```python
from build123d import *

# Parameters (mm, degrees)
SKETCH1_W           = 9.8806
SKETCH1_H           = 5.7658
BOSS_EXTRUDE1_DEPTH = 6.985
SKETCH2_W           = 0.6604
SKETCH2_H           = 0.6604
BOSS_EXTRUDE2_DEPTH = 3.175
SKETCH4_W           = 8.6106
SKETCH4_H           = 4.4958
CUT_EXTRUDE1_DEPTH  = 6.35
SKETCH2_2_W         = 0.6604
SKETCH2_2_H         = 0.6604
BOSS_EXTRUDE3_DEPTH = 6.35
SKETCH5_W           = 0.635
SKETCH5_H           = 1.016
SKETCH5_W_2         = 1.524
SKETCH5_H_2         = 0.635
CUT_EXTRUDE2_DEPTH  = 3.556


with BuildPart() as part:
    # Sketch1 → Boss-Extrude1 (new body)
    with BuildSketch(Plane.XY):
        with Locations((4.9403, 2.8829)):
            Rectangle(SKETCH1_W, SKETCH1_H)
    extrude(amount=BOSS_EXTRUDE1_DEPTH)

    # Sketch2 → Boss-Extrude2 (add)
    with BuildSketch(Plane(origin=(0, 0, 0), x_dir=(-1, 0, 0), z_dir=(0, 0, -1))):
        with Locations((-7.4403, 3.4036)):
            Rectangle(SKETCH2_W, SKETCH2_H)
        with Locations((-4.9403, 3.4036)):
            Rectangle(SKETCH2_W, SKETCH2_H)
        with Locations((-2.4403, 3.4036)):
            Rectangle(SKETCH2_W, SKETCH2_H)
    extrude(amount=BOSS_EXTRUDE2_DEPTH)

    # Sketch4 → Cut-Extrude1 (cut)
    with BuildSketch(Plane.XY.offset(6.985)):
        with Locations((4.9403, 2.8829)):
            Rectangle(SKETCH4_W, SKETCH4_H)
    extrude(amount=-CUT_EXTRUDE1_DEPTH, mode=Mode.SUBTRACT)

    # Sketch2<2> → Boss-Extrude3 (add)
    with BuildSketch(Plane(origin=(0, 0, 0), x_dir=(-1, 0, 0), z_dir=(0, 0, -1))):
        with Locations((-7.4403, 3.4036)):
            Rectangle(SKETCH2_2_W, SKETCH2_2_H)
        with Locations((-4.9403, 3.4036)):
            Rectangle(SKETCH2_2_W, SKETCH2_2_H)
        with Locations((-2.4403, 3.4036)):
            Rectangle(SKETCH2_2_W, SKETCH2_2_H)
    extrude(amount=-BOSS_EXTRUDE3_DEPTH)

    # Sketch5 → Cut-Extrude2 (cut)
    with BuildSketch(Plane.XY.offset(6.985)):
        with Locations((0.3175, 4.3688)):
            Rectangle(SKETCH5_W, SKETCH5_H)
        with Locations((9.5631, 4.3688)):
            Rectangle(SKETCH5_W, SKETCH5_H)
        with Locations((7.2263, 5.4483)):
            Rectangle(SKETCH5_W_2, SKETCH5_H_2)
        with Locations((2.6543, 5.4483)):
            Rectangle(SKETCH5_W_2, SKETCH5_H_2)
    extrude(amount=-CUT_EXTRUDE2_DEPTH, mode=Mode.SUBTRACT)


solid = part.part
```
Geometry: final body of the model. Coordinates: model frame, mm. A direction names the side the tool comes from. Coordinates: 2 decimals unless noted, no trailing zeros. Order: outer loops, then holes, each group sorted by start corner. A loop starts at its lowest first (then second) coordinate and runs counter-clockwise, first axis right, second up. Notation, with made-up numbers: (35.25, -29.75) -> (92.25, -29.75) arc R10 ccw to (92.25, -25.75) -> close; hole circle Ø7 at (41, 33). An arc over 180 degrees is marked (long way). Write item = value, one per line.
(1) Cut plane D-D on x = 3. Return loops of the section in (y, z) (3 decimals), plus the area to 3 significant figures.
Solved:
outline = (0, 0) -> (5.766, 0) -> (5.766, 3.429) -> (5.131, 3.429) -> (5.131, 0.635) -> (0.635, 0.635) -> (0.635, 6.985) -> (0, 6.985) -> close
area = 9.47 mm²
(2) Line query: line 1 (Y direction, x = 7.25, z = 1) (3 decimals); line 2 (X direction, y = 3.7, z = 3) (1 decimal); line 3 (X direction, y = 5, z = 5) (3 decimals). Output: solid intervals per line, ascending.
Solved:
line_1 = 0 to 0.635, 3.073 to 3.734, 5.131 to 5.766
line_2 = 0 to 0.6, 2.1 to 2.8, 4.6 to 5.3, 7.1 to 7.8, 9.2 to 9.9
line_3 = 0 to 0.635, 9.246 to 9.881
(3) Access query for faces 5 (the flat face through (0.635, 3, 4)), 6 (the flat face through (0, 3, 3)). Directions: +Z, -Z, +X, -X, +Y, -Y. A direction counts if a zero-diameter tool reaches every point of the face in a straight line with its end or side. Return the directions, or none.
Solved:
face_5 = +Z
face_6 = +Z, -Z, -X, +Y, -Y
(4) Cut plane A-A on z = -0.5. Return loops of the section in (x, y), plus the area to 3 significant figures.
Solved:
outline = (2.11, 3.07) -> (2.77, 3.07) -> (2.77, 3.73) -> (2.11, 3.73) -> close; (4.61, 3.07) -> (5.27, 3.07) -> (5.27, 3.73) -> (4.61, 3.73) -> close; (7.11, 3.07) -> (7.77, 3.07) -> (7.77, 3.73) -> (7.11, 3.73) -> close
area = 1.31 mm²
(5) Pin query (flat end, axial travel): pin 1 Ø0.5 at (x, z) = (2.5, 4.5) entering from +Y; pin 2 Ø0.5 at (x, y) = (5, 3.5) entering from +Z; pin 3 Ø0.7 at (y, z) = (3.5, -1) entering from -X. Return the tip coordinate at first contact, or that it passes through.
Solved:
pin_1 = 3.73
pin_2 = 6.35
pin_3 = 2.11
(6) Cut plane B-B on z = 3. Return loops of the section in (x, y) (1 decimal), plus the area to 3 significant figures.
Solved:
outline = (0, 0) -> (9.9, 0) -> (9.9, 5.8) -> (0, 5.8) -> close; (2.1, 3.1) -> (2.8, 3.1) -> (2.8, 3.7) -> (2.1, 3.7) -> close; (4.6, 3.1) -> (5.3, 3.1) -> (5.3, 3.7) -> (4.6, 3.7) -> close; (7.1, 3.1) -> (7.8, 3.1) -> (7.8, 3.7) -> (7.1, 3.7) -> close; hole (0.6, 0.6) -> (9.2, 0.6) -> (9.2, 5.1) -> (0.6, 5.1) -> close
area = 19.6 mm²
(7) Cut plane C-C on y = 2.9. Return loops of the section in (x, z) (3 decimals), plus the area to 3 significant figures.
Solved:
outline = (0, 0) -> (9.881, 0) -> (9.881, 6.985) -> (9.246, 6.985) -> (9.246, 0.635) -> (0.635, 0.635) -> (0.635, 6.985) -> (0, 6.985) -> close
area = 14.3 mm²
(8) Pull-direction query (Y, two-part tool) for faces 1 (the flat face through (5, 5.131, 3)), 2 (the flat face through (5, 0, 3)), 3 (the flat face through (5, 5.766, 3)), 4 (the flat face through (8.9, 5.4, 6.985)); classes: pulls with the +Y half, pulls with the -Y half, needs draft (parallel to the pull), parting line crosses it, or undercut.
Solved:
face_1 = undercut
face_2 = pulls with the -Y half
face_3 = pulls with the +Y half
face_4 = needs draft
